from build123d import *

# Parameters (mm, degrees)
F0_W     = 65
F0_H     = 45
F1_DEPTH = 25
F3_D     = 5
F3_DEPTH = 12
F3_TIP   = 1.5021515476
F4_R     = 13
F5_DEPTH = 25.001


with BuildPart() as f1:
    # F0 (on Front) → F1 (new body)
    with BuildSketch(Plane.XZ):
        with Locations((-1.1299671605, -0.7227190264)):
            Rectangle(F0_W, F0_H)
    extrude(amount=F1_DEPTH)

    # F3
    with Locations(Plane.XZ.offset(25)):
        with Locations((-18.0727501515, 0)):
            Hole(F3_D / 2, depth=F3_DEPTH)
            with Locations((0, 0, -(F3_DEPTH + F3_TIP / 2))):  # 118° drill point
                Cone(0, F3_D / 2, F3_TIP, mode=Mode.SUBTRACT)

    # F4 (on face) → F5 (cut, through all)
    with BuildSketch(Plane.XZ.offset(25)):
        with Locations((10.6912245974, -0.0869205323)):
            Circle(F4_R)
    extrude(amount=-F5_DEPTH, mode=Mode.SUBTRACT)


solid = f1.part
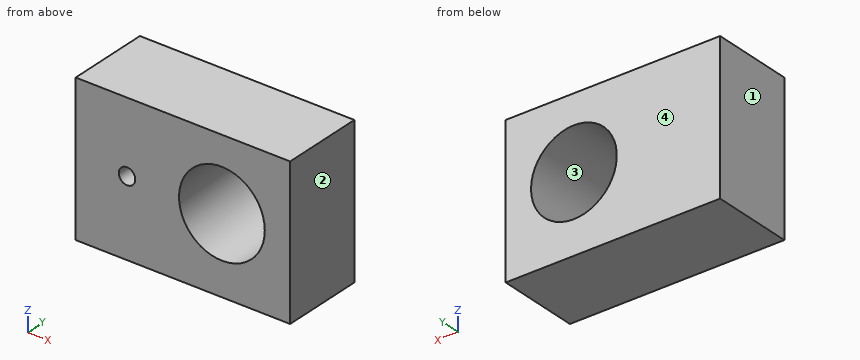
Input: part model. Units: mm. Frame: model coordinates. Face numbers are marked on the shaded views. Round coordinates to 2 decimals unless told otherwise and drop trailing zeros. Write each loop counter-clockwise with the first axis right and the second up, starting at its lowest first coordinate (ties: lowest second). Pieces come first, ordered by that corner, then holes.
1) Cut plane D-D (y = -6). Return the cut outline in (x, z).
2) Contact query for flat-ended pins moving along their axis: P1, Ø15.5, axis at x = 10.69, z = -0.09, coming from the +Y side; P2, Ø6, axis at x = 22, z = 13.5, coming from the +Y side; P3, Ø4, axis at x = -18.07, z = 0, coming from the -Y side. Output: stop coordinate, or through.
3) Cut plane A-A (z = 10). Return the cut outline in (x, y).
4) Cut plane B-B (x = 9). Return the cut outline in (y, z), then the cut area to 3 significant figures.
5) Cut plane C-C (y = -17). Return the cut outline in (x, z).
6) Draft query along X for the marked faces 1, 2, 3 and 4. Return one class per face: pulls with the +X half, pulls with the -X half, needs draft (parallel to the pull), parting line crosses it, or undercut.
7) Ray query, L1, parallel to X at y = -19, z = 0; L2, parallel to Z at x = 11, y = -22; L3, parallel to Z at x = 22.5, y = -7.25. Return the intervals inside material, ascending.
Geometry says:
1. outline: (-33.63, -23.22) - (31.37, -23.22) - (31.37, 21.78) - (-33.63, 21.78) - close; hole circle Ø26 at (10.69, -0.09)
2. P1: passes through
2. P2: stops at y = 0
2. P3: stops at y = -12.7
3. outline: (-33.63, -25) - (2.49, -25) - (2.49, 0) - (-33.63, 0) - close; (18.89, -25) - (31.37, -25) - (31.37, 0) - (18.89, 0) - close
4. outline: (-25, -23.22) - (0, -23.22) - (0, -12.98) - (-25, -12.98) - close; (-25, 12.8) - (0, 12.8) - (0, 21.78) - (-25, 21.78) - close
4. area: 481 mm2
5. outline: (-33.63, -23.22) - (31.37, -23.22) - (31.37, 21.78) - (-33.63, 21.78) - close; hole circle Ø5 at (-18.07, 0); hole circle Ø26 at (10.69, -0.09)
6. face 1: pulls with the -X half
6. face 2: pulls with the +X half
6. face 3: undercut
6. face 4: needs draft
7. L1: x = -33.63 to -20.57, -15.57 to -2.31, 23.69 to 31.37
7. L2: z = -23.22 to -13.08, 12.91 to 21.78
7. L3: z = -23.22 to -5.52, 5.35 to 21.78
